Answer from the drawing. Dimensions are ordinates in mm from the lowest x, y and z of the part. A direction names the side the tool comes from. Coordinates: 2 decimals unless noted, no trailing zeros. Write each loop counter-clockwise with the first axis right and the second up, starting at its lowest first coordinate (ties: lowest second). Pieces come first, ordered by that corner, then holes. Notation, with made-up numbers: (-35.75, 88.5) -> (10.25, 88.5) arc R31 cw to (10.25, 120.5) -> close; hole circle Ø8 at (74, 89). An arc over 180 degrees is marked (long way). Use CSV: the item, a comma, the result in double quotes.
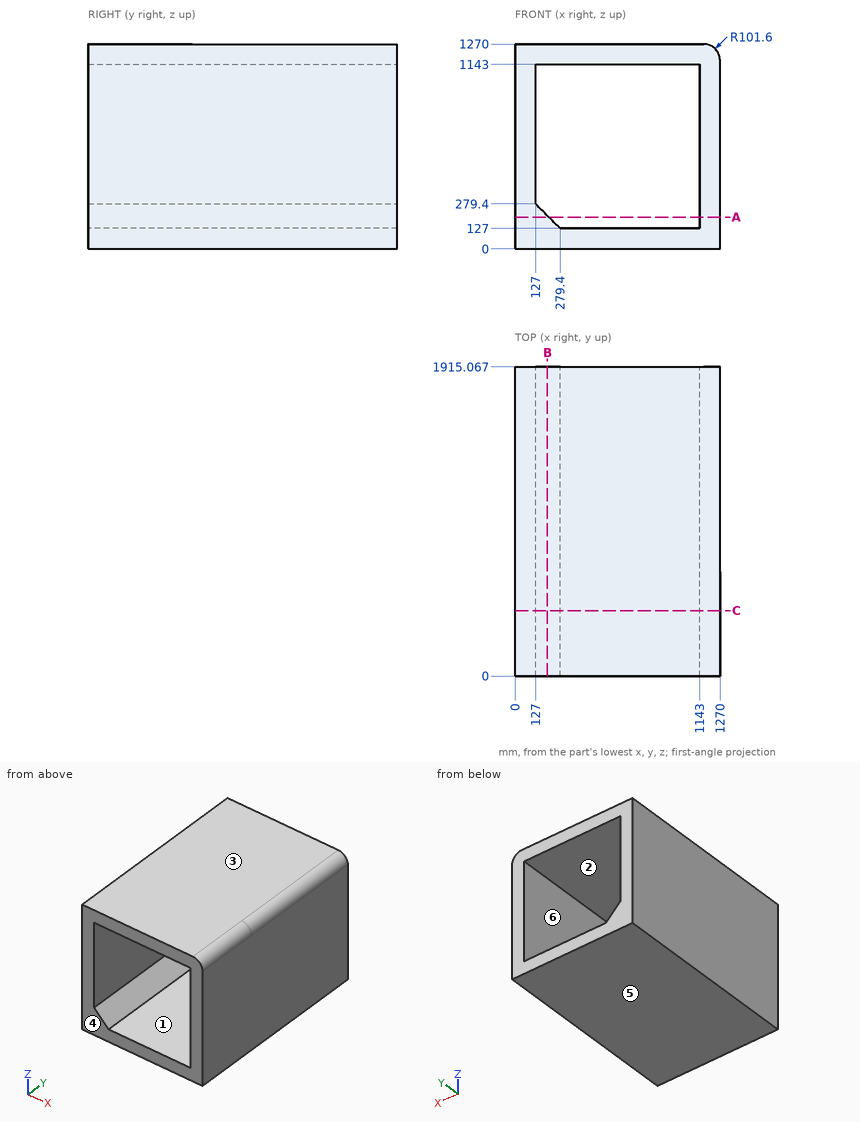
1. This flat-tipped pin is pushed along its axis until it touches: pin 1 Ø2 at (x, y) = (356.5, 503.5) entering from -Z. Where does it stop, or does it pass through?
Solutions:
pin 1,"stops at z = 0"
2. Find the intervals of material crossed by line 1 along Z through (x, y) = (958, 852); line 2 along Z through (x, y) = (273, 1601), in increasing order.
Solutions:
line 1,"z = 0 to 127, 1143 to 1270"
line 2,"z = 0 to 133.4, 1143 to 1270"
3. A cutting plane is placed at C-C (y = 405). Give the vertices of the cut face in (x, z).
Solutions:
outline,"(0, 0) -> (1270, 0) -> (1270, 1168.4) arc R101.6 ccw to (1168.4, 1270) -> (0, 1270) -> close; hole (127, 279.4) -> (279.4, 127) -> (1143, 127) -> (1143, 1143) -> (127, 1143) -> close"
4. A cutting plane is placed at A-A (z = 196.5). Give the vertices of the cut face in (x, y), and give its area (3 significant figures).
Solutions:
outline,"(0, 0) -> (209.9, 0) -> (209.9, 1915.07) -> (0, 1915.07) -> close; (1143, 0) -> (1270, 0) -> (1270, 1915.07) -> (1143, 1915.07) -> close"
area,"645,000 mm^2"
5. For a pull along Z with two mould halves and no side action, classify the marked faces 1, 2, 3 and 4 as pulls with the +Z half, pulls with the -Z half, needs draft (parallel to the pull), parting line crosses it, or undercut.
Solutions:
face 1,"undercut"
face 2,"undercut"
face 3,"pulls with the +Z half"
face 4,"needs draft"
6. A cutting plane is placed at B-B (x = 200.5). Give the vertices of the cut face in (y, z).
Solutions:
outline,"(0, 0) -> (1915.07, 0) -> (1915.07, 205.9) -> (0, 205.9) -> close; (0, 1143) -> (1915.07, 1143) -> (1915.07, 1270) -> (0, 1270) -> close"
7. A tool of negligible diameter and unlimited length cuts with its end or side. For the marked faces 5 and 6, from which of +Z, -Z, +X, -X, +Y, -Y can it reach the whole face along a straight path? Write none if from no direction.
Solutions:
face 5,"-Z, +X, -X, +Y, -Y"
face 6,"+Y, -Y"
